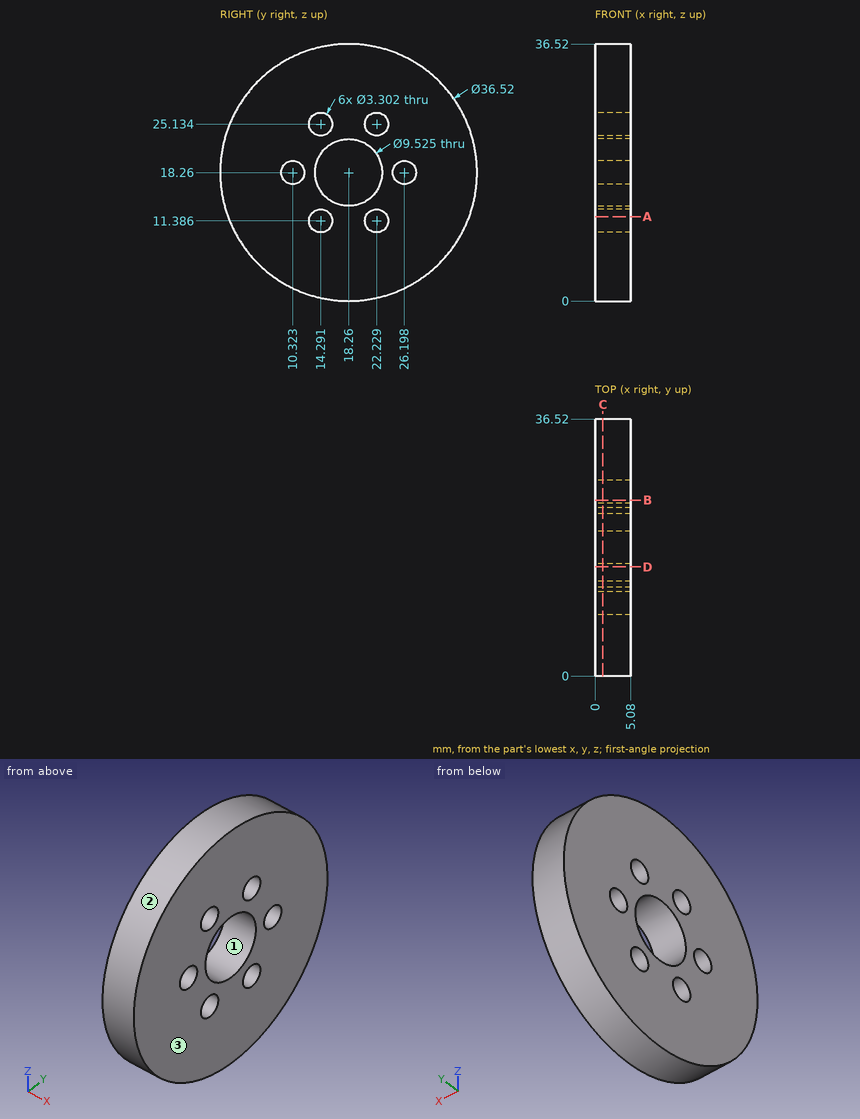
Print and shaded views of the part. All mm, measured from the part's lowest x, y and z. Give positions to 0.01 mm unless a question says otherwise; leave off trailing zeros. Write each loop counter-clockwise with the first axis right and the second up, starting at its lowest first coordinate (ties: lowest second). Pieces come first, ordered by that corner, then holes. Notation, with made-up numbers: (55.5, -22) -> (72.5, -22) arc R21 cw to (72.5, -8) -> close; hole circle Ø8 at (-36.5, 3). An arc over 180 degrees is marked (long way). Write item = value, one per line.
(1) Slice it at C-C, the plane x = 1.1. Give the cut face in (y, z) (1 decimal), then the cut area to 3 significant figures.
Determined:
outline = circle Ø36.5 at (18.3, 18.3); hole circle Ø3.3 at (10.3, 18.3); hole circle Ø3.3 at (14.3, 11.4); hole circle Ø3.3 at (14.3, 25.1); hole circle Ø9.5 at (18.3, 18.3); hole circle Ø3.3 at (22.2, 11.4); hole circle Ø3.3 at (22.2, 25.1); hole circle Ø3.3 at (26.2, 18.3)
area = 925 mm2
(2) Flat gauge pins, fed straight in: P1, Ø2, axis at x = 1, y = 21.5, coming from the -Z side; P2, Ø3, axis at x = 4, y = 10, coming from the +Z side; P3, Ø8, axis at y = 5, z = 21, coming from the -X side; P4, Ø3, axis at x = 3.5, z = 12, coming from the +Y side. Where does each tip first touch, or does it go through?
Determined:
P1 = 0.14
P2 = 35.22
P3 = 0
P4 = 35.89
(3) Probe line 1 along Z through (x, y) = (4.7, 15.5); line 2 along Z through (x, y) = (2.65, 14) (1 decimal); line 3 along Y through (x, z) = (2.1, 17.5) (1 decimal). List the from-to ranges inside material, lowest first.
Determined:
line_1 = 0.21 to 10.26, 12.51 to 14.38, 22.14 to 24.01, 26.26 to 36.31
line_2 = 0.5 to 9.8, 13 to 16.1, 20.4 to 23.5, 26.8 to 36
line_3 = 0 to 8.9, 11.8 to 13.6, 23 to 24.7, 27.7 to 36.5
(4) Slice it at B-B, the plane y = 25. Give the cut face in (x, z).
Determined:
outline = (0, 1.29) -> (5.08, 1.29) -> (5.08, 17.12) -> (0, 17.12) -> close; (0, 19.4) -> (5.08, 19.4) -> (5.08, 35.23) -> (0, 35.23) -> close
(5) Slice it at A-A, the plane z = 12. Give the cut face in (x, y), then the cut area to 3 significant figures.
Determined:
outline = (0, 1.11) -> (5.08, 1.11) -> (5.08, 12.76) -> (0, 12.76) -> close; (0, 15.82) -> (5.08, 15.82) -> (5.08, 20.7) -> (0, 20.7) -> close; (0, 23.76) -> (5.08, 23.76) -> (5.08, 35.41) -> (0, 35.41) -> close
area = 143 mm2
(6) Mould opens along Z. For the marked faces 1, 2 and 3 say: released by +Z, released by -Z, zero draft, split by the parting line, or undercut.
Determined:
face_1 = undercut
face_2 = split by the parting line
face_3 = zero draft
(7) Slice it at D-D, the plane y = 15.5. Give the cut face in (x, z), then the cut area to 3 significant figures.
Determined:
outline = (0, 0.21) -> (5.08, 0.21) -> (5.08, 10.26) -> (0, 10.26) -> close; (0, 12.51) -> (5.08, 12.51) -> (5.08, 14.38) -> (0, 14.38) -> close; (0, 22.14) -> (5.08, 22.14) -> (5.08, 24.01) -> (0, 24.01) -> close; (0, 26.26) -> (5.08, 26.26) -> (5.08, 36.31) -> (0, 36.31) -> close
area = 121 mm2
